Design review of the part built by this model. Coordinates are the model's own, in mm. A direction names the side the tool comes from. Give positions to 0.01 mm unless a question says otherwise; leave off trailing zeros. Order: outer loops, then holes, each group sorted by start corner. A loop starts at its lowest first (then second) coordinate and runs counter-clockwise, first axis right, second up.
```python
from build123d import *

# Parameters (mm, degrees)
F1_DEPTH  = 8
F2_R      = 3.25
F2_R_2    = 12.5
F3_DEPTH  = 10
F4_W      = 20
F4_H      = 10
F5_DEPTH  = 30
F7_DEPTH  = 63
F9_DEPTH  = 4
F11_DEPTH = 7
F13_D     = 6.5
F13_DEPTH = 15
F13_TIP   = 1.9527970118
F15_DEPTH = 63
F17_DEPTH = 8
F19_DEPTH = 8


# Not quite as in the source:
# - a pattern or mirror of a feature is missing from the dataset's text; its kind, count and spacing are read off the source's solid


with BuildPart() as f1:
    # F0 (on Top) → F1 (new body)
    with BuildSketch(Plane.XY):
        Polygon((76.5, 31.5), (-76.5, 31.5), (-76.5, -31.5), (76.5, -31.5), (101.5, -31.5), (101.5, 31.5), align=None)
    extrude(amount=F1_DEPTH)

    # F2 (on face) → F3 (join)
    with BuildSketch(Plane(origin=(-76.5, 0, 0), x_dir=(0, -1, 0), z_dir=(-1, 0, 0))):
        with BuildLine():
            Line((31.5, 8), (31.5, 39.5))
            ThreePointArc((31.5, 39.5), (0, 71), (-31.5, 39.5))
            Line((-31.5, 39.5), (-31.5, 8))
            Line((-31.5, 8), (31.5, 8))
        make_face()
        with Locations((-17.6776695297, 21.8223304703)):
            Circle(F2_R, mode=Mode.SUBTRACT)
        with Locations((17.6776695297, 21.8223304703)):
            Circle(F2_R, mode=Mode.SUBTRACT)
        with Locations((0, 39.5)):
            Circle(F2_R_2, mode=Mode.SUBTRACT)
        with Locations((-17.6776695297, 57.1776695297)):
            Circle(F2_R, mode=Mode.SUBTRACT)
        with Locations((17.6776695297, 57.1776695297)):
            Circle(F2_R, mode=Mode.SUBTRACT)
    extrude(amount=-F3_DEPTH)

    # F4 (on face) → F5 (join)
    with BuildSketch(Plane.XY.offset(8)):
        with Locations((43.5, 13.5)):
            Rectangle(F4_W, F4_H)
        with Locations((43.5, -16.5)):
            Rectangle(F4_W, F4_H)
    extrude(amount=F5_DEPTH)

    # F6 (on face) → F7 (join)
    with BuildSketch(Plane.XY.offset(8)):
        Polygon((97.5, 13.5), (101.5, 13.5), (101.5, 31.5), (94.5, 31.5), (94.5, 16.5), (97.5, 16.5), align=None)
        Polygon((94.5, -31.5), (101.5, -31.5), (101.5, -16.5), (97.5, -16.5), (97.5, -19.5), (94.5, -19.5), align=None)
    extrude(amount=F7_DEPTH)

    # F8 (on face) → F9 (join, through all)
    with BuildSketch(Plane.YZ.offset(101.5)):
        Polygon((13.5, 71), (-16.5, 71), (-16.5, 46), (-1.5, 56), (13.5, 46), align=None)
    extrude(amount=-F9_DEPTH)

    # F10 (on face) → F11 (join)
    with BuildSketch(Plane.XZ.offset(31.5)):
        Polygon((89.5, 8), (94.5, 13), (94.5, 20.0710678119), (85.9644660941, 11.5355339059), (82.4289321881, 8), align=None)
    f11 = extrude(amount=-F11_DEPTH)

    # F11_copies: F11 across plane
    add(f11.mirror(Plane.ZX))

    # F13
    with Locations(Plane.YZ.offset(101.5)):
        with Locations((-24.5, 63), (24.5, 63), (24.5, 30), (-24.5, 30)):
            Hole(F13_D / 2, depth=F13_DEPTH)
            with Locations((0, 0, -(F13_DEPTH + F13_TIP / 2))):  # 118° drill point
                Cone(0, F13_D / 2, F13_TIP, mode=Mode.SUBTRACT)

    # F14 (on face) → F15 (join)
    with BuildSketch(Plane.XZ.offset(31.5)):
        Polygon((-66.5, 13), (-66.5, 8), (-61.5, 8), align=None)
    extrude(amount=-F15_DEPTH)

    # F16 (on face) → F17 (cut)
    with BuildSketch(Plane.XY.offset(8)):
        with BuildLine():
            ThreePointArc((-24.5, 22), (-22, 24.5), (-24.5, 27))
            Line((-24.5, 27), (-31.5, 27))
            ThreePointArc((-31.5, 27), (-34, 24.5), (-31.5, 22))
            Line((-31.5, 22), (-24.5, 22))
        make_face()
        with BuildLine():
            ThreePointArc((3.5, 22), (6, 24.5), (3.5, 27))
            Line((3.5, 27), (-3.5, 27))
            ThreePointArc((-3.5, 27), (-6, 24.5), (-3.5, 22))
            Line((-3.5, 22), (3.5, 22))
        make_face()
        with BuildLine():
            ThreePointArc((3.5, -27), (6, -24.5), (3.5, -22))
            Line((3.5, -22), (-3.5, -22))
            ThreePointArc((-3.5, -22), (-6, -24.5), (-3.5, -27))
            Line((-3.5, -27), (3.5, -27))
        make_face()
        with BuildLine():
            ThreePointArc((-24.5, -27), (-22, -24.5), (-24.5, -22))
            Line((-24.5, -22), (-31.5, -22))
            ThreePointArc((-31.5, -22), (-34, -24.5), (-31.5, -27))
            Line((-31.5, -27), (-24.5, -27))
        make_face()
    extrude(amount=-F17_DEPTH, mode=Mode.SUBTRACT)

    # F18 (on face) → F19 (cut)
    with BuildSketch(Plane.XY.offset(8)):
        Polygon((-49.5, 16.5), (-52.3867513459, 16.5), (-55.2735026919, 11.5), (-49.5, 11.5), align=None)
        Polygon((-46.6132486541, 16.5), (-49.5, 16.5), (-49.5, 11.5), (-55.2735026919, 11.5), (-52.3867513459, 6.5), (-46.6132486541, 6.5), (-43.7264973081, 11.5), align=None)
        Polygon((-42.3724755983, 4.0214471492), (-45.2592269442, -0.9785528508), (-42.3724755983, -5.9785528508), (-36.5989729064, -5.9785528508), (-33.7122215604, -0.9785528508), (-36.5989729064, 4.0214471492), align=None)
        Polygon((-31.3867513459, 16.5), (-34.2735026919, 11.5), (-31.3867513459, 6.5), (-25.6132486541, 6.5), (-22.7264973081, 11.5), (-25.6132486541, 16.5), align=None)
        Polygon((-21.3724755983, 4.0214471492), (-24.2592269442, -0.9785528508), (-21.3724755983, -5.9785528508), (-15.5989729064, -5.9785528508), (-12.7122215604, -0.9785528508), (-15.5989729064, 4.0214471492), align=None)
        Polygon((-10.3867513459, 16.5), (-13.2735026919, 11.5), (-10.3867513459, 6.5), (-4.6132486541, 6.5), (-1.7264973081, 11.5), (-4.6132486541, 16.5), align=None)
        Polygon((-0.3724755983, 4.0214471492), (-3.2592269442, -0.9785528508), (-0.3724755983, -5.9785528508), (5.4010270936, -5.9785528508), (8.2877784396, -0.9785528508), (5.4010270936, 4.0214471492), align=None)
        Polygon((10.6132486541, 16.5), (7.7264973081, 11.5), (10.6132486541, 6.5), (16.3867513459, 6.5), (19.2735026919, 11.5), (16.3867513459, 16.5), align=None)
        Polygon((20.6275244017, 4.0214471492), (17.7407730558, -0.9785528508), (20.6275244017, -5.9785528508), (26.4010270936, -5.9785528508), (29.2877784396, -0.9785528508), (26.4010270936, 4.0214471492), align=None)
        Polygon((-52.4131430724, -8.4999860695), (-55.2998944183, -13.4999860695), (-52.4131430724, -18.4999860695), (-46.6396403805, -18.4999860695), (-43.7528890345, -13.4999860695), (-46.6396403805, -8.4999860695), align=None)
        Polygon((-31.4131430724, -8.4999860695), (-34.2998944183, -13.4999860695), (-31.4131430724, -18.4999860695), (-25.6396403805, -18.4999860695), (-22.7528890345, -13.4999860695), (-25.6396403805, -8.4999860695), align=None)
        Polygon((-10.4131430724, -8.4999860695), (-13.2998944183, -13.4999860695), (-10.4131430724, -18.4999860695), (-4.6396403805, -18.4999860695), (-1.7528890345, -13.4999860695), (-4.6396403805, -8.4999860695), align=None)
        Polygon((10.5868569276, -8.4999860695), (7.7001055817, -13.4999860695), (10.5868569276, -18.4999860695), (16.3603596195, -18.4999860695), (19.2471109655, -13.4999860695), (16.3603596195, -8.4999860695), align=None)
        Polygon((77.7407730558, -0.9785528508), (80.6275244017, -5.9785528508), (86.4010270936, -5.9785528508), (89.2877784396, -0.9785528508), (86.4010270936, 4.0214471492), (80.6275244017, 4.0214471492), align=None)
        Polygon((79.2471109655, -13.4999860695), (76.3603596195, -8.4999860695), (70.5868569276, -8.4999860695), (67.7001055817, -13.4999860695), (70.5868569276, -18.4999860695), (76.3603596195, -18.4999860695), align=None)
        Polygon((76.3867513459, 16.5), (70.6132486541, 16.5), (67.7264973081, 11.5), (70.6132486541, 6.5), (76.3867513459, 6.5), (79.2735026919, 11.5), align=None)
        Polygon((68.2877784396, -0.9785528508), (65.4010270936, 4.0214471492), (59.6275244017, 4.0214471492), (56.7407730558, -0.9785528508), (59.6275244017, -5.9785528508), (65.4010270936, -5.9785528508), align=None)
        Polygon((37.7407730558, -0.9785528508), (40.6275244017, -5.9785528508), (46.4010270936, -5.9785528508), (49.2877784396, -0.9785528508), (46.4010270936, 4.0214471492), (40.6275244017, 4.0214471492), align=None)
    extrude(amount=-F19_DEPTH, mode=Mode.SUBTRACT)


solid = f1.part
```
1. Machinability: for faces 4 (the face through (43, 18.5, 23)), 5 (the face through (-28, -27, 4)), 6 (the face through (53.5, 13, 23)), 7 (the face through (43, 8.5, 23)), which of the approach directions +Z, -Z, +X, -X, +Y, -Y give a long, thin tool a straight path to every point of the face, cutting with its end or side? Answer none if there is none.
Recorded:
face 4: +Z, +Y
face 5: +Z, -Z
face 6: +Z, +Y, -Y
face 7: +Z, +X
2. Take a section at C-C (z = 30). State how many separate pieces and enclosed holes the cut face has, then the cut area to 3 significant figures.
Recorded:
separate pieces: 8
enclosed holes: 0
area: 990 mm2
3. For pin 1 (5 mm diameter, centred on x = 44.5, y = -19, fed in from +Z); pin 2 (4 mm diameter, centred on y = 16.5, z = 22, fed in from -X); pin 3 (10 mm diameter, centred on x = 40.5, z = 26, fed in from -Y), all flat-tipped, find the tip position at first contact; note any pin that passes through.
Recorded:
pin 1: stops at z = 38
pin 2: stops at x = 33.5
pin 3: stops at y = -21.5
4. Draft analysis for pull direction Z (two halves, no side actions). For faces 1 (the face through (97.951, 26.895, 65.197)), 2 (the face through (43, -16, 38)), 3 (the face through (-22.84, -3.44, 4.06)), state which applies: pulls with the +Z half, pulls with the -Z half, needs draft (parallel to the pull), parting line crosses it, or undercut.
Recorded:
face 1: undercut
face 2: pulls with the +Z half
face 3: needs draft
5. Take a section at B-B (z = 63). State the section outline as (x, y) points, then the cut area to 3 significant figures.
Recorded:
outline: (-76.5, -20.98) - (-66.5, -20.98) - (-66.5, 20.98) - (-76.5, 20.98) - close; (94.5, -31.5) - (101.5, -31.5) - (101.5, -27.75) - (94.5, -27.75) - close; (94.5, -21.25) - (101.5, -21.25) - (101.5, 21.25) - (94.5, 21.25) - (94.5, 16.5) - (97.5, 16.5) - (97.5, -19.5) - (94.5, -19.5) - close; (94.5, 27.75) - (101.5, 27.75) - (101.5, 31.5) - (94.5, 31.5) - close
area: 662 mm2
6. Take a section at A-A (x = 74.5). State the section outline as (y, z) points, then the cut area to 3 significant figures.
Recorded:
outline: (-31.5, 0) - (-18.5, 0) - (-18.5, 8) - (-31.5, 8) - close; (-8.5, 0) - (6.5, 0) - (6.5, 8) - (-8.5, 8) - close; (16.5, 0) - (31.5, 0) - (31.5, 8) - (16.5, 8) - close
area: 344 mm2
7. For line 1 along Z through (x, y) = (96, -24); line 2 along X through (y, z) = (11, 64); line 3 along X through (y, z) = (-25.5, 46), list the stretches that pass through material, from the lowest coordinate up.
Recorded:
line 1: z = 0 to 26.79, 33.21 to 59.79, 66.21 to 71
line 2: x = -76.5 to -66.5, 97.5 to 101.5
line 3: x = -76.5 to -66.5, 94.5 to 101.5
